Model file for the job. Use its own axes, mm. Face numbers are marked on the shaded views. A direction names the side the tool comes from. Round coordinates to 2 decimals unless told otherwise and drop trailing zeros. Loops run counter-clockwise (first coordinate to the right, second up) from the corner with the lowest first, then second, coordinate; pieces in that order, holes last. Notation, with made-up numbers: (-5.5, -22) -> (3.5, -22) arc R18 ccw to (3.5, -7) -> close; hole circle Ø8 at (26.25, 71.5). An arc over 180 degrees is marked (long way). Use a Markdown table: item, result. Add a question column.
```python
from build123d import *

# Parameters (mm, degrees)
PAD_DEPTH       = 12.5
PAD001_DEPTH    = 10
POCKET_DEPTH    = 199.738093
SKETCH003_R     = 3.25
POCKET001_DEPTH = 10


with BuildPart() as part:
    # Sketch → Pad (new body, symmetric)
    with BuildSketch(Plane.XY):
        with BuildLine():
            ThreePointArc((0, -20), (20, 0), (0, 20))
            Line((0, 25), (0, 20))
            ThreePointArc((0, -25), (25, 0), (0, 25))
            Line((0, -20), (0, -25))
        make_face()
    extrude(amount=PAD_DEPTH, both=True)

    # Sketch001 → Pad001 (join, symmetric)
    with BuildSketch(Plane.XY):
        with BuildLine():
            Line((0, 25), (0, 40))
            Line((0, 40), (10, 40))
            Line((10, 40), (28, 22))
            Line((28, 22), (28, -22))
            Line((28, -22), (10, -40))
            Line((10, -40), (0, -40))
            Line((0, -40), (0, -25))
            ThreePointArc((0, -25), (25, 0), (0, 25))
        make_face()
    extrude(amount=PAD001_DEPTH, both=True)

    # Sketch002 (on DatumPlane) → Pocket (cut, through all)
    with BuildSketch(Plane.YZ.offset(5)):
        with BuildLine():
            ThreePointArc((32.5, 6), (26.5, 0), (32.5, -6))
            Line((113.900581, -6), (32.5, -6))
            Line((113.900581, 6), (113.900581, -6))
            Line((32.5, 6), (113.900581, 6))
        make_face()
    pocket = extrude(amount=POCKET_DEPTH, mode=Mode.SUBTRACT)

    # Mirrored: Pocket across XZ
    add(pocket.mirror(Plane.XZ), mode=Mode.SUBTRACT)

    # Sketch003 (on DatumPlane) → Pocket001 (cut)
    with BuildSketch(Plane.YZ.offset(5)):
        with Locations((32.5, 0)):
            Circle(SKETCH003_R)
        with Locations((-32.5, 0)):
            Circle(SKETCH003_R)
    extrude(amount=-POCKET001_DEPTH, mode=Mode.SUBTRACT)


solid = part.part
```
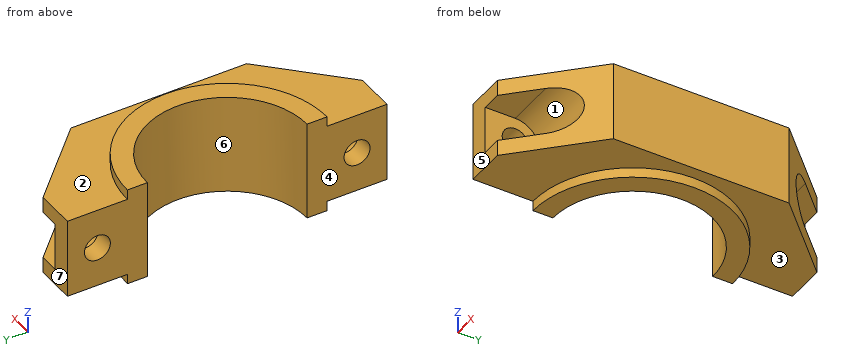
1) Cut at B-B on y = 0. Write the cut outline in (x, z), and give its area (3 significant figures).
2) Cut at C-C on x = 6.75. Write the cut outline in (y, z), and give its area (3 significant figures).
3) Pull direction Y, two halves, no side cores. Call the marked faces 5, 6 and 7: +Y half, -Y half, draft (parallel to the pull), parting line (faces both ways), or undercut.
4) Pin check, flat tips, straight feed: pin 1 Ø6 at (y, z) = (4.5, -2.5) entering from -X; pin 2 Ø13 at (y, z) = (32, 0) entering from +X; pin 3 Ø4 at (x, y) = (13, -37) entering from -Z. Stop position of each tip, or through.
5) Wall check: probe 1 along Z at (x, y) = (2.3, -32.5); probe 2 along Y at (x, z) = (25, -1.5); probe 3 along X at (y, z) = (-26.5, -5). Give the ranges that are in metal, low to high. Write a range as from..to.
6) Cut at A-A on z = 0. Write the cut outline in (x, y), and give its area (3 significant figures).
7) Cut at D-D on z = 7.25. Write the cut outline in (x, y), and give its area (3 significant figures).
8) Tool access for the marked faces 1, 2, 3 and 4: list every direction of +Z, -Z, +X, -X, +Y, -Y with a clear straight run to the whole face (end or side of a thin tool).
Established:
| question | item | result |
|---|---|---|
| 1 | outline | (20, -12.5) -> (25, -12.5) -> (25, -10) -> (28, -10) -> (28, 10) -> (25, 10) -> (25, 12.5) -> (20, 12.5) -> close |
| 1 | area | 185 mm^2 |
| 2 | outline | (-40, -10) -> (-24.07, -10) -> (-24.07, -12.5) -> (-18.83, -12.5) -> (-18.83, 12.5) -> (-24.07, 12.5) -> (-24.07, 10) -> (-40, 10) -> (-40, 6) -> (-32.5, 6) arc R6 cw to (-32.5, -6) -> (-40, -6) -> close; (18.83, -12.5) -> (24.07, -12.5) -> (24.07, -10) -> (40, -10) -> (40, -6) -> (32.5, -6) arc R6 cw to (32.5, 6) -> (40, 6) -> (40, 10) -> (24.07, 10) -> (24.07, 12.5) -> (18.83, 12.5) -> close |
| 2 | area | 606 mm^2 |
| 3 | face 5 | -Y half |
| 3 | face 6 | undercut |
| 3 | face 7 | +Y half |
| 4 | pin 1 | stops at x = 18.54 |
| 4 | pin 2 | stops at x = 24.5 |
| 4 | pin 3 | stops at z = -10 |
| 5 | probe 1 | z = -10..-3.25, 3.25..10 |
| 5 | probe 2 | y = -25..25 |
| 5 | probe 3 | x = 0..23.5 |
| 6 | outline | (0, -40) -> (5, -40) -> (5, -35.75) -> (0, -35.75) -> close; (0, -29.25) -> (5, -29.25) -> (5, -26.5) -> (23.5, -26.5) -> (28, -22) -> (28, 22) -> (23.5, 26.5) -> (5, 26.5) -> (5, 29.25) -> (0, 29.25) -> (0, 20) arc R20 cw to (0, -20) -> close; (0, 35.75) -> (5, 35.75) -> (5, 40) -> (0, 40) -> close |
| 6 | area | 905 mm^2 |
| 7 | outline | (0, -40) -> (10, -40) -> (28, -22) -> (28, 22) -> (10, 40) -> (0, 40) -> (0, 20) arc R20 cw to (0, -20) -> close |
| 7 | area | 1,290 mm^2 |
| 8 | face 1 | +X, -Y |
| 8 | face 2 | +Z, +X |
| 8 | face 3 | -Z, +X |
| 8 | face 4 | +Z, -Z, -X, +Y, -Y |
